Design review of the part built by this model. Coordinates are the model's own, in mm. Coordinates: 2 decimals unless noted, no trailing zeros. Write each loop counter-clockwise with the first axis right and the second up, starting at its lowest first coordinate (ties: lowest second). Pieces come first, ordered by that corner, then holes. Notation, with made-up numbers: (-39, 10.5) - (-24, 10.5) arc R15 ccw to (-24, 15.5) - close; hole circle Ø10 at (17.25, 22.25). An arc over 180 degrees is marked (long way). Use a Markdown table: item, result.
from build123d import *

# Parameters (mm, degrees)
F0_W     = 290
F0_H     = 250
F1_DEPTH = 20
F2_SIZE  = 19.99999
F3_SIZE  = 5


# Not quite as in the source:
# - a fillet or chamfer is up to 0.001 mm smaller than in the source, because OpenCascade refuses the exact size


with BuildPart() as f1:
    # F0 (on Top) → F1 (new body)
    with BuildSketch(Plane.XY):
        Rectangle(F0_W, F0_H)
    extrude(amount=F1_DEPTH)

    # F2 (size 20 in the source; OpenCascade refuses exactly that, so slightly less here)
    f2_edges = [f1.edges().sort_by_distance(p)[0] for p in [
        (0, 125, 0),
    ]]
    chamfer(f2_edges, length=F2_SIZE)

    # F3
    f3_edges = [f1.edges().sort_by_distance(p)[0] for p in [
        (0, -125, 20),
        (0, -125, 0),
        (145, 0, 20),
        (145, -125, 10),
        (-145, -125, 10),
        (-145, 0, 20),
    ]]
    chamfer(f3_edges, length=F3_SIZE)


solid = f1.part
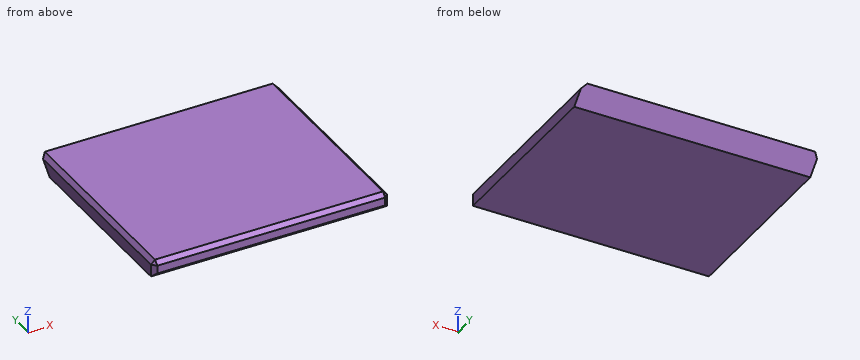
(1) For pin 1 (8 mm diameter, centred on x = -78, z = 10.5, fed in from +Y); pin 2 (5 mm diameter, centred on x = -1.5, z = 14.5, fed in from +Y), all flat-tipped, find the tip position at first contact; note any pin that passes through.
Determined:
| item | result |
|---|---|
| pin 1 | y = 119.5 |
| pin 2 | y = 122 |
(2) For L1, parallel to Y at x = -89.5, z = 4.5; L2, parallel to Y at x = 71, z = 15; L3, parallel to X at y = 105.5, z = 17, list the stretches that pass through material, from the lowest coordinate up. Write a range as from..to.
Determined:
| item | result |
|---|---|
| L1 | -124.5..109.5 |
| L2 | -125..120 |
| L3 | -143..143 |
(3) Take a section at B-B on z = 9.25. Write out the cut boundary in (x, y).
Determined:
| item | result |
|---|---|
| outline | (-145, -120) - (-140, -125) - (140, -125) - (145, -120) - (145, 114.25) - (-145, 114.25) - close |
